Autodesk Inventor part; units mm, degrees
ref_plane "Work Plane1" through (-48.25, 120.3736, 22.5) normal (0, 0, -1) x (0, 1, 0)
ref_plane "YZ Plane" through (0, 0, 0) normal (1, 0, 0) x (0, 1, 0)
ref_plane "XZ Plane" through (0, 0, 0) normal (0, 1, 0) x (-1, 0, 0)
sketch "Sketch1" plane through (0, 0, 0) normal (0, 0, 1) x (1, 0, 0)
  circle A0 centre (-88.75, 237.1618) radius 2
  circle A1 centre (-45.25, 302.7734) radius 2
  circle A2 centre (-88.75, 302.7734) radius 2
  circle A3 centre (-45.25, 237.1618) radius 2
  circle A4 centre (-46.75, 361.06) radius 2
  circle A5 centre (-40.75, 400) radius 23.3333
  line L0 (-53.25, 186.7791) -> (-53.25, -39)
  arc A6 (-53.25, -39) -> (-46.25, -46) centre (-46.25, -39) ccw
  line L1 (1.25, -46) -> (-46.25, -46)
  arc A7 (1.25, -46) -> (8.9167, 45.3566) centre (1.25, 0) ccw
  arc A8 (7.25, 47.3286) -> (8.9167, 45.3566) centre (9.25, 47.3286) ccw
  line L2 (7.25, 400) -> (7.25, 47.3286)
  arc A9 (7.25, 400) -> (-27.0387, 446) centre (-40.75, 400) ccw
  line L3 (-85.75, 446) -> (-27.0387, 446)
  circle A10 centre (-85.75, 438.7) radius 2
  circle A11 centre (-85.75, 361.06) radius 2
  circle A12 centre (-46.75, 438.7) radius 2
  circle A13 centre (10.9583, -29.879) radius 2.1
  circle A14 centre (32.6667, 0) radius 2.1
  circle A15 centre (-24.1666, -18.4663) radius 2.1
  circle A16 centre (10.9583, 29.879) radius 2.1
  circle A17 centre (-24.1666, 18.4663) radius 2.1
  circle A18 centre (1.25, 0) radius 23.3333
  circle A19 centre (-1.75, 302.7734) radius 2.25
  circle A20 centre (-1.75, 237.1618) radius 2.25
  circle A21 centre (-43.75, 127.6736) radius 2
  circle A22 centre (-4.75, -38.7) radius 2
  circle A23 centre (-4.75, 38.94) radius 2
  circle A24 centre (-4.75, 127.6736) radius 2
  circle A25 centre (-43.75, -38.7) radius 2
  circle A26 centre (-43.75, 38.94) radius 2
  line L4 (-88.75, 237.1618) -> (-95.75, 237.1618)
  line L5 (-1.75, 237.1618) -> (5.25, 237.1618)
  circle A27 centre (-88.75, 237.1618) radius 7
  circle A28 centre (-1.75, 237.1618) radius 7
  line L6 (-88.75, 230.1618) -> (-1.75, 230.1618)
  line L7 (-88.75, 244.1618) -> (-1.75, 244.1618)
  circle A29 centre (-9.3333, 400) radius 2.1
  circle A30 centre (-31.0417, 429.879) radius 2.1
  circle A31 centre (-31.0417, 370.121) radius 2.1
  circle A32 centre (-66.1666, 418.4663) radius 2.1
  circle A33 centre (-66.1666, 381.5337) radius 2.1
  arc A34 (-95.75, 226.7791) -> (-85.75, 216.7791) centre (-85.75, 226.7791) ccw
  line L8 (-85.75, 216.7791) -> (-83.25, 216.7791)
  arc A35 (-53.25, 186.7791) -> (-83.25, 216.7791) centre (-83.25, 186.7791) ccw
  arc A36 (-85.75, 446) -> (-95.75, 436) centre (-85.75, 436) ccw
  line L9 (-95.75, 226.7791) -> (-95.75, 436)
  point P0 (0, 0)
  dimension "d0" = 7
  dimension "d1" = 7
ref_plane "Work Plane1" through (-48.25, 120.3736, 22.5) normal (0, 0, -1) x (0, 1, 0)
extrude "Extrusion1" add sketch "Sketch1" along normal up to surface (22.5 mm away) contours A27 | L7 A28 L6 A27 | A28
sketch "Sketch2" plane through (-88.75, 230.1618, 0) normal (0, -1, 0) x (1, 0, 0)
  circle A0 centre (22.5, 22.5) radius 16
  circle A1 centre (64.5, 22.5) radius 16
  line L0 (0, 22.5) -> (87, 22.5)
  line L1 (0, 0) -> (0, 22.5)
  line L2 (0, 0) -> (87, 0)
  line L3 (87, 0) -> (87, 22.5)
  point P0 (88.75, 0)
  point P1 (80.5, 22.5)
  point P2 (48.5, 22.5)
  point P3 (38.5, 22.5)
  point P4 (6.5, 22.5)
extrude "Extrusion2" cut sketch "Sketch2" against normal through all contours A0 L0 | L0 A1 picked at (22.9879, 15.9292) picked at (60.5079, 16.4106)
properties part number "Uchwyt_silnika_podwojny"
The listing builds one solid part. Answer for the finished solid, in the listing's coordinates (mm). Coordinates: 2 decimals unless noted, no trailing zeros. Order: outer loops, then holes, each group sorted by start corner. A loop starts at its lowest first (then second) coordinate and runs counter-clockwise, first axis right, second up.
Q1. A cutting plane is placed at C-C, the plane y = 231. Write down the section's boundary in (x, z).
Q2. Given P1, Ø1, axis at x = -11, y = 242, coming from the +Z side; P2, Ø1.5, axis at x = -57.5, y = 242.5, coming from the +Z side, each flat-ended and moving along its own axis, determine where each tip first touches the part or whether it passes through.
Q3. A cutting plane is placed at B-B, the plane z = 12.5. Write down the section's boundary in (x, y), and give its area (3 significant figures).
Q4. For a pull along Y with two mould halves and no side action, classify faces 1 (the face through (-46, 244.162, 9)), 2 (the face through (-45.51, 235.18, 11.09)), 3 (the face through (-46, 240, 0)) as pulls with the +Y half, pulls with the -Y half, needs draft (parallel to the pull), parting line crosses it, or undercut.
Q5. A cutting plane is placed at A-A, the plane x = -45.25. Write down the section's boundary in (y, z), and give its area (3 significant figures).
Q6. A cutting plane is placed at D-D, the plane z = 2.75. Write down the section's boundary in (x, y).
Q7. Consider line 1 (Y direction, x = -45.25, z = 11.5); line 2 (X direction, y = 235.5, z = 20); line 3 (X direction, y = 231, z = 21.25). Determine where each line is inside the solid, lowest interval first.
Answers follow:
1. outline: (-92.07, 0) - (1.57, 0) - (1.57, 22.5) - (-8.25, 22.5) arc R16 cw to (-40.25, 22.5) - (-50.25, 22.5) arc R16 cw to (-82.25, 22.5) - (-92.07, 22.5) - close
2. P1: stops at z = 14.32
2. P2: stops at z = 9.63
3. outline: (-88.75, 230.16) - (-78.74, 230.16) - (-78.74, 244.16) - (-88.75, 244.16) arc R7 ccw to start; (-53.76, 230.16) - (-36.74, 230.16) - (-36.74, 244.16) - (-53.76, 244.16) - close; (-11.76, 230.16) - (-1.75, 230.16) arc R7 ccw to (-1.75, 244.16) - (-11.76, 244.16) - close; hole circle Ø4 at (-88.75, 237.16); hole circle Ø4 at (-45.25, 237.16); hole circle Ø4.5 at (-1.75, 237.16)
3. area: 631 mm2
4. face 1: pulls with the +Y half
4. face 2: undercut
4. face 3: needs draft
5. outline: (230.16, 0) - (235.16, 0) - (235.16, 22.5) - (230.16, 22.5) - close; (239.16, 0) - (244.16, 0) - (244.16, 22.5) - (239.16, 22.5) - close
5. area: 225 mm2
6. outline: (-88.75, 230.16) - (-1.75, 230.16) arc R7 ccw to (-1.75, 244.16) - (-88.75, 244.16) arc R7 ccw to start; hole circle Ø4 at (-88.75, 237.16); hole circle Ø4 at (-45.25, 237.16); hole circle Ø4.5 at (-1.75, 237.16)
7. line 1: y = 230.16 to 235.16, 239.16 to 244.16
7. line 2: x = -95.55 to -89.86, -87.64 to -82.05, -50.45 to -46.36, -44.14 to -40.05, -8.45 to -3.27, -0.23 to 5.05
7. line 3: x = -92.07 to -82.2, -50.3 to -40.2, -8.3 to 1.57
